Geometry check sheet. Reference: the model listing, model coordinates, mm. Round coordinates to 2 decimals unless told otherwise and drop trailing zeros. Order: outer loops, then holes, each group sorted by start corner. A loop starts at its lowest first (then second) coordinate and runs counter-clockwise, first axis right, second up.
```python
from build123d import *

# Parameters (mm, degrees)
SKETCH1_R           = 3.175
SKETCH1_R_2         = 12.954
SKETCH1_R_3         = 31.877
BOSS_EXTRUDE1_DEPTH = 2.54


with BuildPart() as part:
    # Sketch1 → Boss-Extrude1 (new body)
    with BuildSketch(Plane(origin=(0, 0, 0), x_dir=(1, 0, 0), z_dir=(0, 1, 0))):
        with BuildLine():
            Line((96.26346, 21.909734203), (16.385721429, 48.755177759))
            ThreePointArc((16.385721429, 48.755177759), (0, 51.435), (-16.385721429, 48.755177759))
            Line((-16.385721429, 48.755177759), (-96.26346, 21.909734203))
            ThreePointArc((-96.26346, 21.909734203), (-112.014, 0), (-96.26346, -21.909734203))
            Line((-96.26346, -21.909734203), (-16.385721429, -48.755177759))
            ThreePointArc((-16.385721429, -48.755177759), (0, -51.435), (16.385721429, -48.755177759))
            Line((16.385721429, -48.755177759), (96.26346, -21.909734203))
            ThreePointArc((96.26346, -21.909734203), (112.014, 0), (96.26346, 21.909734203))
        make_face()
        with Locations(Location((-41.275, 0, 0), (0, 0, 270))):
            Circle(SKETCH1_R, mode=Mode.SUBTRACT)
        with Locations(Location((0, -41.275, 0), (0, 0, 270))):
            Circle(SKETCH1_R, mode=Mode.SUBTRACT)
        with Locations(Location((-88.9, 0, 0), (0, 0, 270))):
            Circle(SKETCH1_R_2, mode=Mode.SUBTRACT)
        with Locations(Location((0, 0, 0), (0, 0, 270))):
            Circle(SKETCH1_R_3, mode=Mode.SUBTRACT)
        with Locations(Location((41.275, 0, 0), (0, 0, 270))):
            Circle(SKETCH1_R, mode=Mode.SUBTRACT)
        with Locations(Location((88.9, 0, 0), (0, 0, 270))):
            Circle(SKETCH1_R_2, mode=Mode.SUBTRACT)
        with Locations(Location((0, 41.275, 0), (0, 0, 270))):
            Circle(SKETCH1_R, mode=Mode.SUBTRACT)
    extrude(amount=BOSS_EXTRUDE1_DEPTH)


solid = part.part
```
(1) Material ranges on line 1 (X direction, y = 0.4, z = 10); line 2 (X direction, y = 2.2, z = 5.5); line 3 (Z direction, x = 2, y = 0.2), recorded low to high.
Returned:
line 1: x = -109.74 to -97.13, -80.67 to -30.27, 30.27 to 80.67, 97.13 to 109.74
line 2: x = -111.35 to -100.63, -77.17 to -31.4, 31.4 to 77.17, 100.63 to 111.35
line 3: z = -51.4 to -43.74, -38.81 to -31.81, 31.81 to 38.81, 43.74 to 51.4
(2) Sectioned sample at D-D, the plane x = -92. Record the cut outline in (y, z), and give its area (3 significant figures).
Returned:
outline: (0, -23.34) - (2.54, -23.34) - (2.54, -12.58) - (0, -12.58) - close; (0, 12.58) - (2.54, 12.58) - (2.54, 23.34) - (0, 23.34) - close
area: 54.7 mm2
(3) Sectioned sample at A-A, the plane z = 0. Record the cut outline in (x, y), and give its area (3 significant figures).
Returned:
outline: (-112.01, 0) - (-101.85, 0) - (-101.85, 2.54) - (-112.01, 2.54) - close; (-75.95, 0) - (-44.45, 0) - (-44.45, 2.54) - (-75.95, 2.54) - close; (-38.1, 0) - (-31.88, 0) - (-31.88, 2.54) - (-38.1, 2.54) - close; (31.88, 0) - (38.1, 0) - (38.1, 2.54) - (31.88, 2.54) - close; (44.45, 0) - (75.95, 0) - (75.95, 2.54) - (44.45, 2.54) - close; (101.85, 0) - (112.01, 0) - (112.01, 2.54) - (101.85, 2.54) - close
area: 243 mm2
(4) Draft check along X on faces 1 (the flat face through (55.77, 1.25, 35.52)), 2 (the cylindrical face through (31.606, 1.252, -4.15)), 3 (the cylindrical face through (43.95, 1.25, 1.71)), 4 (the cylindrical face through (-112.01, 1.25, -0.4)). Enter one of: released by +X, released by -X, zero draft, split by the parting line, or undercut.
Returned:
face 1: released by +X
face 2: undercut
face 3: undercut
face 4: released by -X
(5) Sectioned sample at B-B, the plane x = 0. Record the cut outline in (y, z) (3 decimals).
Returned:
outline: (0, -51.435) - (2.54, -51.435) - (2.54, -44.45) - (0, -44.45) - close; (0, -38.1) - (2.54, -38.1) - (2.54, -31.877) - (0, -31.877) - close; (0, 31.877) - (2.54, 31.877) - (2.54, 38.1) - (0, 38.1) - close; (0, 44.45) - (2.54, 44.45) - (2.54, 51.435) - (0, 51.435) - close
(6) Sectioned sample at C-C, the plane y = 1.4. Record the cut outline in (x, z) (3 decimals), and give its area (3 significant figures).
Returned:
outline: (-96.263, -21.91) - (-16.386, -48.755) arc R51.435 ccw to (16.386, -48.755) - (96.263, -21.91) arc R23.114 ccw to (96.263, 21.91) - (16.386, 48.755) arc R51.435 ccw to (-16.386, 48.755) - (-96.263, 21.91) arc R23.114 ccw to start; hole circle Ø25.908 at (-88.9, 0); hole circle Ø6.35 at (-41.275, 0); hole circle Ø63.754 at (0, 0); hole circle Ø6.35 at (0, -41.275); hole circle Ø6.35 at (0, 41.275); hole circle Ø6.35 at (41.275, 0); hole circle Ø25.908 at (88.9, 0)
area: 11,200 mm2
